```python
from build123d import *

# Parameters (mm, degrees)
ESBO_O2_OUTSIDE_W          = 42.476
ESBO_O2_OUTSIDE_H          = 42.476
ESBO_O2_OUTSIDE_W_2        = 28
ESBO_O2_OUTSIDE_H_2        = 15
CORTE_EXTRUS_O1_DEPTH      = 25.1
CORTE_EXTRUS_O1_DEPTH_BACK = 25.1
CORTE_EXTRUS_O2_DEPTH      = 16


with BuildPart() as part:
    # Esboço1 one side → Revolução1 (revolve)
    with BuildSketch(Plane.XY):
        with BuildLine():
            ThreePointArc((4, 23.516407865), (2.02117415, 23.953333716), (0, 24.1))
            Line((0, 24.1), (0, -24.1))
            ThreePointArc((0, -24.1), (2.02117415, -23.953333716), (4, -23.516407865))
            Line((4, -23.516407865), (14, -10.1))
            Line((14, -10.1), (9.9, -10.1))
            Line((9.9, -10.1), (9.9, 10.1))
            Line((9.9, 10.1), (14, 10.1))
            Line((14, 10.1), (4, 23.516407865))
        make_face()
    revolve(axis=Axis((0, -24.1, 0), (0, 1, 0)))

    # Esboço2 outside → Corte-extrusão1 (cut, two sides)
    with BuildSketch(Plane(origin=(0, 0, 0), x_dir=(1, 0, 0), z_dir=(0, 1, 0))) as corte_extrus_o1_sk:
        Rectangle(ESBO_O2_OUTSIDE_W, ESBO_O2_OUTSIDE_H)
        Rectangle(ESBO_O2_OUTSIDE_W_2, ESBO_O2_OUTSIDE_H_2, mode=Mode.SUBTRACT)
    extrude(amount=CORTE_EXTRUS_O1_DEPTH, mode=Mode.SUBTRACT)
    extrude(corte_extrus_o1_sk.sketch, amount=-CORTE_EXTRUS_O1_DEPTH_BACK, mode=Mode.SUBTRACT)

    # Esboço3 → Corte-extrusão2 (cut, through all)
    with BuildSketch(Plane(origin=(0, 0, -7.5), x_dir=(-1, 0, 0), z_dir=(0, 0, -1))):
        with BuildLine():
            Line((6, 24.1), (6, 8.6))
            ThreePointArc((6, 8.6), (0, 2.6), (-6, 8.6))
            Line((-6, 8.6), (-6, 24.1))
            ThreePointArc((-6, 24.1), (0, 30.1), (6, 24.1))
        make_face()
        with BuildLine():
            Line((-6, -24.1), (-6, -8.6))
            ThreePointArc((-6, -8.6), (0, -2.6), (6, -8.6))
            Line((6, -8.6), (6, -24.1))
            ThreePointArc((6, -24.1), (0, -30.1), (-6, -24.1))
        make_face()
    extrude(amount=-CORTE_EXTRUS_O2_DEPTH, mode=Mode.SUBTRACT)


solid = part.part
```
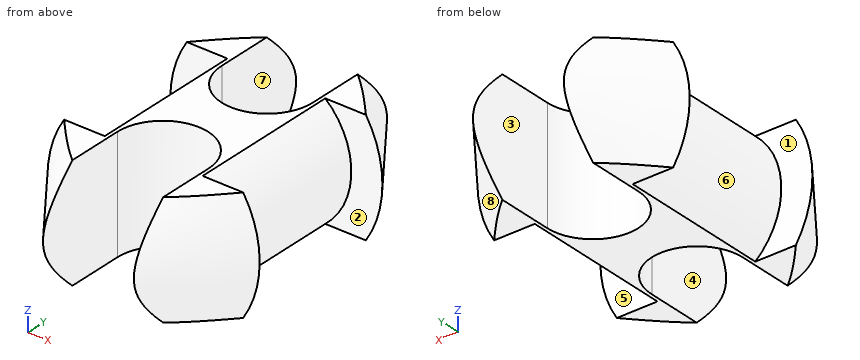
Source: CAD feature listing. Evaluate the final solid. Frame: model axes, mm. Face numbers are marked on the shaded views. A direction names the side the tool comes from. Coordinates: 2 decimals unless noted, no trailing zeros. Write each loop counter-clockwise with the first axis right and the second up, starting at its lowest first coordinate (ties: lowest second). Pieces come first, ordered by that corner, then holes. Notation, with made-up numbers: (71.5, 54.25) - (97.5, 54.25) arc R26 cw to (97.5, 77.25) - close; hole circle Ø9 at (14.25, 75.25). An arc over 180 degrees is marked (long way). Answer as a JSON object with one key per item and string values.
Q1. First-contact query: pin 1 Ø6 at (y, z) = (13.5, 3) entering from +X (3 decimals); pin 2 Ø4 at (x, z) = (-12, 1.5) entering from -Y; pin 3 Ø6 at (x, z) = (11.5, -0.5) entering from -Y. Flat tips, straight axial feed; report the tip coordinate or a pass-through.
Ans:
{"pin 1": "stops at x = 13.445", "pin 2": "stops at y = -15.34", "pin 3": "stops at y = -17.46"}
Q2. Section query B-B, the plane y = 12.5. Output: boundary loops of the cut face in (x, z), plus the area to 3 significant figures.
Ans:
{"outline": "(-9.64, -7.5) - (-6, -7.5) - (-6, 7.5) - (-9.64, 7.5) arc R12.21 ccw to start; (6, -7.5) - (9.64, -7.5) arc R12.21 ccw to (9.64, 7.5) - (6, 7.5) - close", "area": "162 mm2"}
Q3. Material intervals for line 1 (Y direction, x = 9.5, z = -7); line 2 (X direction, y = 17, z = 3); line 3 (X direction, y = 16, z = 3), sorted ascending. Write a range as [from, to].
Ans:
{"line 1": "y = [-13.05, -10.1], [10.1, 13.05]", "line 2": "x = [-8.33, -6], [6, 8.33]", "line 3": "x = [-9.12, -6], [6, 9.12]"}
Q4. Section query A-A, the plane y = 6. Output: boundary loops of the cut face in (x, z).
Ans:
{"outline": "(-6.46, -7.5) - (-5.41, -7.5) - (-5.41, 7.5) - (-6.46, 7.5) arc R9.9 ccw to start; (5.41, -7.5) - (6.46, -7.5) arc R9.9 ccw to (6.46, 7.5) - (5.41, 7.5) - close"}
Q5. Section query D-D, the plane x = -3.5. Output: boundary loops of the cut face in (y, z).
Ans:
{"outline": "(-3.73, -7.5) - (3.73, -7.5) - (3.73, 7.5) - (-3.73, 7.5) - close"}
Q6. Draft query along X for the marked faces 5, 6, 7 and 8. Return one class per face: released by +X, released by -X, zero draft, split by the parting line, or undercut.
Ans:
{"face 5": "zero draft", "face 6": "released by -X", "face 7": "undercut", "face 8": "released by +X"}
Q7. Set-up query: the marked faces 1, 2, 3 and 4. Return all of +Z, -Z, +X, -X, +Y, -Y with unobstructed straight access to the full face (end or side cutting, diameter ignored); none if empty.
Ans:
{"face 1": "-X", "face 2": "+X", "face 3": "+Z, -Z, +Y", "face 4": "+Z, -Z, -Y"}
Q8. Section query C-C, the plane x = 0. Output: boundary loops of the cut face in (y, z), plus the area to 3 significant figures.
Ans:
{"outline": "(-2.6, -7.5) - (2.6, -7.5) - (2.6, 7.5) - (-2.6, 7.5) - close", "area": "78.0 mm2"}
